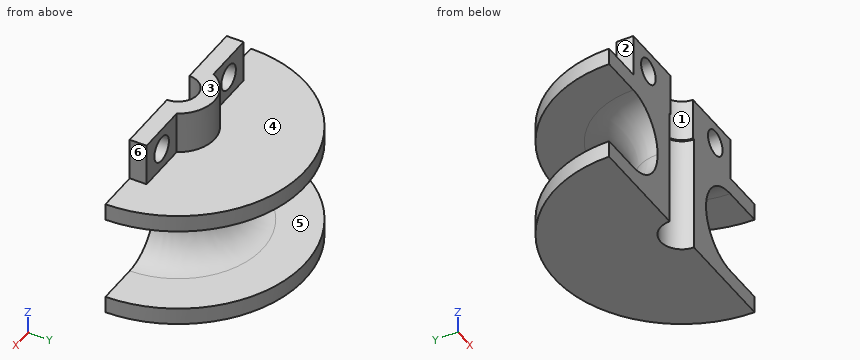
```python
from build123d import *

# Parameters (mm, degrees)
F1_ANGLE = 180
F3_DEPTH = 5
F4_R     = 1.5
F5_DEPTH = 2.001
F6_R     = 4.99999


# Not quite as in the source:
# - a fillet or chamfer is up to 0.001 mm smaller than in the source, because OpenCascade refuses the exact size


with BuildPart() as f1:
    # F0 (on Front) → F1 (revolve)
    with BuildSketch(Plane.XZ):
        Polygon((-2.5, -7), (-2.5, 7), (-15, 7), (-15, 5), (-5, 5), (-5, -5), (-15, -5), (-15, -7), align=None)
    revolve(axis=Axis((0, 0, 0.6770828075), (0, 0, -1)), revolution_arc=F1_ANGLE)

    # F2 (on face) → F3 (join)
    with BuildSketch(Plane.XY.offset(7)):
        with BuildLine():
            Line((-10, 2), (-10, 0))
            Line((-10, 0), (-2.3, 0))
            ThreePointArc((-2.3, 0), (0, 2.3), (2.3, 0))
            Line((2.3, 0), (10, 0))
            Line((10, 0), (10, 2))
            Line((10, 2), (3.8065732621, 2))
            ThreePointArc((3.8065732621, 2), (0, 4.3), (-3.8065732621, 2))
            Line((-3.8065732621, 2), (-10, 2))
        make_face()
    extrude(amount=F3_DEPTH)

    # F4 (on face) → F5 (cut, through all)
    with BuildSketch(Plane(origin=(0, 2, 0), x_dir=(-1, 0, 0), z_dir=(0, 1, 0))):
        with Locations((6.9032866311, 9.5)):
            Circle(F4_R)
        with Locations((-6.9032866311, 9.5)):
            Circle(F4_R)
    extrude(amount=-F5_DEPTH, mode=Mode.SUBTRACT)

    # F6 (radius 5 in the source; OpenCascade refuses exactly that, so slightly less here)
    f6_edges = [f1.edges().sort_by_distance(p)[0] for p in [
        (0, 5, 5),
        (0, 5, -5),
    ]]
    fillet(f6_edges, radius=F6_R)


solid = f1.part
```
Here's how the part is built. I have some questions about the finished solid (model axes, mm). Face numbers are marked on the shaded views. A direction names the side the tool comes from. Coordinates: 2 decimals unless noted, no trailing zeros. Loops run counter-clockwise (first coordinate to the right, second up) from the corner with the lowest first, then second, coordinate; pieces in that order, holes last. Notation, with made-up numbers: (-17.5, -36) - (28.5, -36) arc R24 ccw to (28.5, 3) - close; hole circle Ø2 at (-27, 26). An arc over 180 degrees is marked (long way). Return JSON: item names as keys, results as strings. Group by question number.
Item 1: If we section it at A-A on y = 12: Write out the boundary of the cut face in (x, z), and give its area (3 significant figures).
Item 2: On a 3-axis mill with a long thin cutter (end or side, diameter ignored), from which of +Z, -Z, +X, -X, +Y, -Y can I reach the whole of each face in a straight line? I mean the marked faces 4, 5 and 6. Say none if no direction works.
Item 3: Will these pins go through, and if not, where does the flat tip stop? P1, Ø2.5, axis at x = 6.5, z = 10, coming from the +Y side; P2, Ø8, axis at y = 12.5, z = 9, coming from the -X side; P3, Ø3, axis at x = 4.5, y = 4.5, coming from the +Z side.
Item 4: We'd pull the mould along X, two halves only. Please class the marked faces 1, 2 and 3: +X half, -X half, draft (parallel to the pull), parting line (faces both ways), or undercut.
Item 5: If we section it at C-C on z = 9.5: Write out the boundary of the cut face in (x, y).
Item 6: I need wall thicknesses on line 1 (Z direction, x = -13, y = 4.25); line 2 (Z direction, x = -2.75, y = 5.25); line 3 (Z direction, x = -2, y = 4). Which ranges of each line are inside material? Lowest first, please. Write a range as from..to.
Item 7: If we section it at B-B on x = -11.5: Write out the boundary of the cut face in (y, z), and give its area (3 significant figures).
Calculated:
{
 "1": {"outline": "(-9, -7) - (9, -7) - (9, -5) - (-9, -5) - close; (-9, 5) - (9, 5) - (9, 7) - (-9, 7) - close", "area": "72.0 mm^2"},
 "2": {"face 4": "+Z, +Y", "face 5": "+Y", "face 6": "+Z, +X, +Y, -Y"},
 "3": {"P1": "stops at y = 2", "P2": "stops at x = -11.97", "P3": "stops at z = 7"},
 "4": {"face 1": "undercut", "face 2": "-X half", "face 3": "draft"},
 "5": {"outline": "(-10, 0) - (-8.4, 0) - (-8.4, 2) - (-10, 2) - close; (-5.4, 0) - (-2.3, 0) arc R2.3 cw to (2.3, 0) - (5.4, 0) - (5.4, 2) - (3.81, 2) arc R4.3 ccw to (-3.81, 2) - (-5.4, 2) - close; (8.4, 0) - (10, 0) - (10, 2) - (8.4, 2) - close"},
 "6": {"line 1": "z = -7..-5, 5..7", "line 2": "z = -7..-2.9, 2.9..7", "line 3": "z = -7..7"},
 "7": {"outline": "(0, -7) - (9.63, -7) - (9.63, -5) - (0, -5) - close; (0, 5) - (9.63, 5) - (9.63, 7) - (0, 7) - close", "area": "38.5 mm^2"}
}
